Build history of the part. All positions in model axes, mm. A direction names the side the tool comes from. Give positions to 0.01 mm unless a question says otherwise; leave off trailing zeros. Order: outer loops, then holes, each group sorted by start corner. A loop starts at its lowest first (then second) coordinate and runs counter-clockwise, first axis right, second up. Notation, with made-up numbers: (58.25, -11.75) - (113.25, -11.75) arc R13 cw to (113.25, 0.25) - close; hole circle Ø1 at (69.25, 6.25). An arc over 180 degrees is marked (long way). One line per item, written item: value.
```python
from build123d import *

# Parameters (mm, degrees)
F0_DEPTH       = 44.45
F1_D           = 4.826
F1_CBORE_D     = 8.73125
F1_CBORE_DEPTH = 1.5875


with BuildPart() as f0:
    # F2 (on Front) → F0 (new body, symmetric)
    with BuildSketch(Plane.XZ):
        Polygon((14.2875, 2.38125), (-14.2875, 2.38125), (-14.2875, 0.79375), (-11.1125, -2.38125), (14.2875, -2.38125), align=None)
    extrude(amount=F0_DEPTH, both=True)

    # F1 (through all)
    with Locations(Plane(origin=(0, 0, -2.38125), x_dir=(1, 0, 0), z_dir=(0, 0, -1))):
        with Locations((1.5875, 34.925), (1.5875, -34.925)):
            CounterBoreHole(F1_D / 2, F1_CBORE_D / 2, F1_CBORE_DEPTH)


solid = f0.part
```
(1) Pin check, flat tips, straight feed: P1, Ø11.5, axis at x = 1.59, y = -34.92, coming from the -Z side; P2, Ø4.5, axis at x = 1.59, y = 34.92, coming from the +Z side. Stop position of each tip, or through.
Completed:
P1: z = -2.38
P2: through
(2) Drill centre lines: line 1 (Y direction, x = 4, z = -1.4); line 2 (Y direction, x = -1.25, z = -1); line 3 (Z direction, x = 3, y = 31.5). Where is each one in solid material? Low to high.
Completed:
line 1: -44.45 to -38.56, -31.29 to 31.29, 38.56 to 44.45
line 2: -44.45 to -38.24, -31.61 to 31.61, 38.24 to 44.45
line 3: -0.79 to 2.38
(3) Slice it at C-C, the plane y = -11.5. Give the cut face in (x, z), and give its area (3 significant figures).
Completed:
outline: (-14.29, 0.79) - (-11.11, -2.38) - (14.29, -2.38) - (14.29, 2.38) - (-14.29, 2.38) - close
area: 131 mm²
(4) 3-axis set-ups, long thin cutter, end or side, ignore diameter. For faces 4 (the face through (0, -44.45, 0)), 5 (the face through (0.641, -30.663, -1.599)): which of +Z, -Z, +X, -X, +Y, -Y reach the whole face in a straight line?
Completed:
face 4: +Z, -Z, +X, -X, -Y
face 5: -Z
(5) Slice it at A-A, the plane x = 2.5. Give the cut face in (y, z), and give its area (3 significant figures).
Completed:
outline: (-44.45, -2.38) - (-39.19, -2.38) - (-39.19, -0.79) - (-37.16, -0.79) - (-37.16, 2.38) - (-44.45, 2.38) - close; (-32.69, -0.79) - (-30.66, -0.79) - (-30.66, -2.38) - (30.66, -2.38) - (30.66, -0.79) - (32.69, -0.79) - (32.69, 2.38) - (-32.69, 2.38) - close; (37.16, -0.79) - (39.19, -0.79) - (39.19, -2.38) - (44.45, -2.38) - (44.45, 2.38) - (37.16, 2.38) - close
area: 368 mm²
(6) Slice it at B-B, the plane z = 0. Count the separate pieces of the cut face and the enclosed holes in it, and give its area (3 significant figures).
Completed:
separate pieces: 1
enclosed holes: 2
area: 2,430 mm²
(7) Pull direction X, two halves, no side cores. Call faces 1 (the face through (14.288, -1, 0)), 2 (the face through (1.902, 32.533, 0.816)), 3 (the face through (0, -1, 2.381)): +X half, -X half, draft (parallel to the pull), parting line (faces both ways), or undercut.
Completed:
face 1: +X half
face 2: undercut
face 3: draft
